Drawing for the job (mm, zero at the part's lowest x, y, z). A direction names the side the tool comes from. Give positions to 0.01 mm unless a question says otherwise; leave off trailing zeros. Order: outer loops, then holes, each group sorted by start corner. A loop starts at its lowest first (then second) coordinate and runs counter-clockwise, first axis right, second up. Notation, with made-up numbers: (80, 44) - (124, 44) arc R7 cw to (124, 57) - close; hole circle Ø6 at (40.5, 17.25). An arc over 180 degrees is marked (long way). One line per item, written item: value.
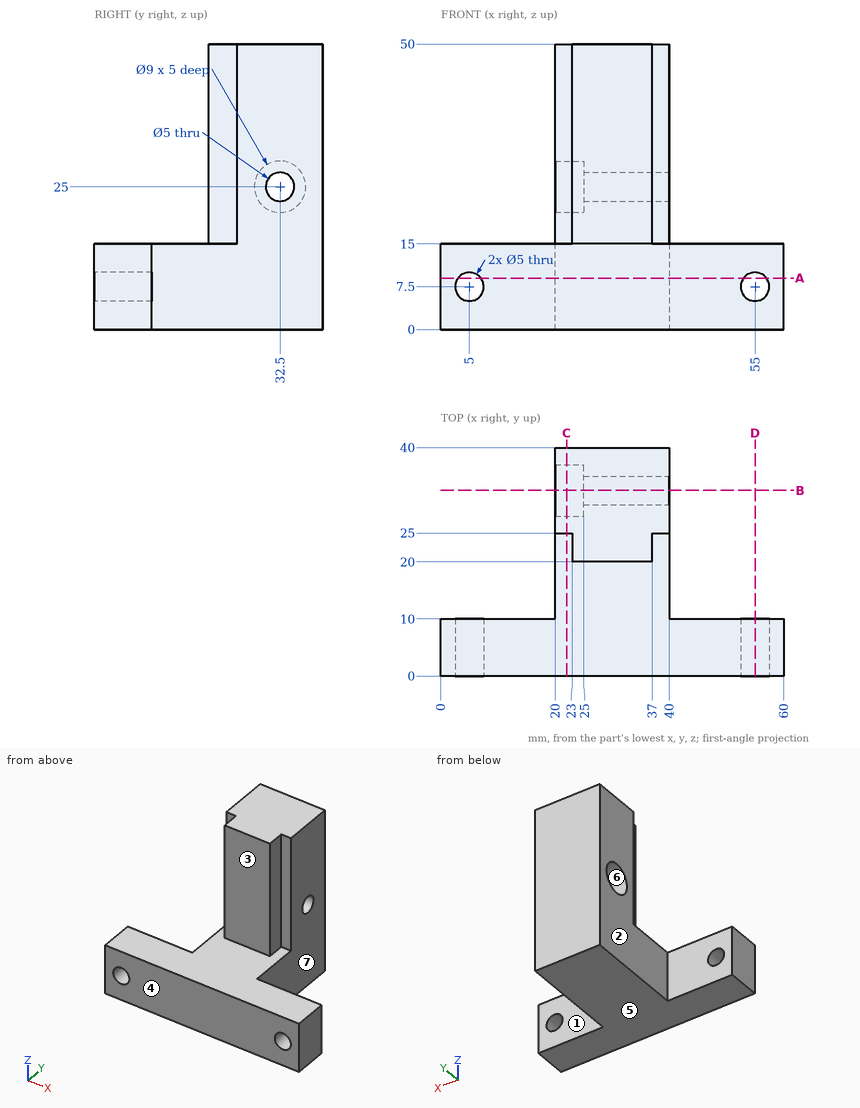
1) Cut at C-C, the plane x = 22. Give the cut face in (y, z), then the cut area to 3 significant figures.
Outcome:
outline: (0, 0) - (40, 0) - (40, 50) - (25, 50) - (25, 15) - (0, 15) - close; hole circle Ø9 at (32.5, 25)
area: 1,060 mm^2
2) Cut at D-D, the plane x = 55. Give the cut face in (y, z).
Outcome:
outline: (0, 0) - (10, 0) - (10, 5) - (0, 5) - close; (0, 10) - (10, 10) - (10, 15) - (0, 15) - close
3) Drill centre lines: line 1 along X through (y, z) = (6.25, 7.5); line 2 along Z through (x, y) = (21.8, 32.5); line 3 along Y through (x, z) = (21, 25). Where is each one in solid material? Low to high. Write a range as from..to.
Outcome:
line 1: x = 0..2.5, 7.5..52.5, 57.5..60
line 2: z = 0..20.5, 29.5..50
line 3: y = 25..28, 37..40
4) Cut at B-B, the plane y = 32.5. Give the cut face in (x, z).
Outcome:
outline: (20, 0) - (40, 0) - (40, 22.5) - (25, 22.5) - (25, 20.5) - (20, 20.5) - close; (20, 29.5) - (25, 29.5) - (25, 27.5) - (40, 27.5) - (40, 50) - (20, 50) - close
5) Mould opens along Z. For the marked faces 5, 6 and 7 say: released by +Z, released by -Z, zero draft, split by the parting line, or undercut.
Outcome:
face 5: released by -Z
face 6: undercut
face 7: zero draft
6) Cut at A-A, the plane z = 9. Give the cut face in (x, y), then the cut area to 3 significant figures.
Outcome:
outline: (0, 0) - (3, 0) - (3, 10) - (0, 10) - close; (7, 0) - (53, 0) - (53, 10) - (40, 10) - (40, 40) - (20, 40) - (20, 10) - (7, 10) - close; (57, 0) - (60, 0) - (60, 10) - (57, 10) - close
area: 1,120 mm^2
7) Which spindle directions (+Z, -Z, +X, -X, +Y, -Y) get a long thin tool onto all of the face, cutting with end or side? Do the marked faces 1, 2, 3 and 4. Say none if no direction does.
Outcome:
face 1: +Z, -Z, +X, +Y
face 2: +Z, -Z, -X, +Y
face 3: +Z, +X, -X, -Y
face 4: +Z, -Z, +X, -X, -Y
8) Pin check, flat tips, straight feed: pin 1 (8 mm diameter, centred on y = 24, z = 41.5, fed in from -X); pin 2 (3.5 mm diameter, centred on x = 39, z = 36.5, fed in from -Y); pin 3 (1.5 mm diameter, centred on y = 21.5, z = 26, fed in from -X). Stop position of each tip, or through.
Outcome:
pin 1: stops at x = 20
pin 2: stops at y = 25
pin 3: stops at x = 23
